Input: part model. Units: mm. Frame: model coordinates. Face numbers are marked on the shaded views. A direction names the side the tool comes from. Round coordinates to 2 decimals unless told otherwise and drop trailing zeros. Loops run counter-clockwise (first coordinate to the right, second up) from the corner with the lowest first, then second, coordinate; pieces in that order, holes last.
1) Access query for the marked faces 4 and 5. Directions: +Z, -Z, +X, -X, +Y, -Y. A direction counts if a zero-diameter tool reaches every point of the face in a straight line with its end or side. Return the directions, or none.
2) Ray query, line 1 along Y through (x, z) = (33, 70); line 2 along X through (y, z) = (22, 67.5); line 3 along Z through (x, y) = (37.5, 10.5). Return the intervals inside material, ascending.
3) Section C-C, the plane y = 71.5. Return loops of the section in (x, z).
4) Section A-A, the plane z = 45.5. Return loops of the section in (x, y), and give its area (3 significant figures).
5) Section B-B, the plane x = 59. Return loops of the section in (y, z).
6) Draft query along Y for the marked faces 1, 2 and 3. Return one class per face: pulls with the +Y half, pulls with the -Y half, needs draft (parallel to the pull), parting line crosses it, or undercut.
7) First-contact query: pin 1 (6 mm diameter, centred on x = 82, y = 57, fed in from +Z). Flat tip, straight axial feed; report the tip coordinate or a pass-through.
from build123d import *

# Parameters (mm, degrees)
SKETCH1_W           = 106.68
SKETCH1_H           = 81.28
BOSS_EXTRUDE1_DEPTH = 81.28
CHAMFER1_SIZE       = 15
SHELL2_T            = -6


with BuildPart() as part:
    # Sketch1 → Boss-Extrude1 (new body)
    with BuildSketch(Plane.XY):
        with Locations((53.34, 40.64)):
            Rectangle(SKETCH1_W, SKETCH1_H)
    extrude(amount=BOSS_EXTRUDE1_DEPTH)

    # Chamfer1
    chamfer1_edges = [part.edges().sort_by_distance(p)[0] for p in [
        (0, 81.28, 40.64),
        (106.68, 0, 40.64),
    ]]
    chamfer(chamfer1_edges, length=CHAMFER1_SIZE)

    # Shell2
    shell2_openings = [part.faces().sort_by_distance(p)[0] for p in [
        (53.34, 40.64, 81.28),
    ]]
    offset(amount=SHELL2_T, openings=shell2_openings, kind=Kind.INTERSECTION)


solid = part.part
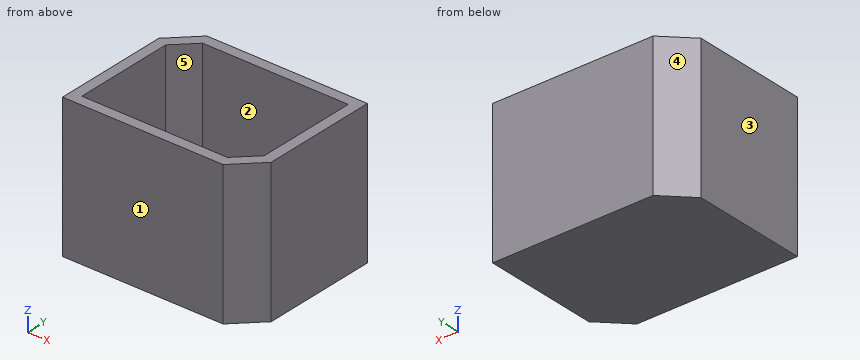
Final values:
1. face 4: +Z, -Z, -X, +Y
1. face 5: +Z
2. line 1: y = 0 to 6, 75.28 to 81.28
2. line 2: x = 0 to 6, 100.68 to 106.68
2. line 3: z = 0 to 6
3. outline: (5.22, 0) - (106.68, 0) - (106.68, 81.28) - (100.68, 81.28) - (100.68, 6) - (13.71, 6) - (13.71, 81.28) - (5.22, 81.28) - close
4. outline: (0, 0) - (91.68, 0) - (106.68, 15) - (106.68, 81.28) - (15, 81.28) - (0, 66.28) - close; hole (6, 6) - (89.19, 6) - (100.68, 17.49) - (100.68, 75.28) - (17.49, 75.28) - (6, 63.79) - close
4. area: 2,020 mm2
5. outline: (0, 0) - (81.28, 0) - (81.28, 81.28) - (75.28, 81.28) - (75.28, 6) - (6, 6) - (6, 81.28) - (0, 81.28) - close
6. face 1: pulls with the -Y half
6. face 2: undercut
6. face 3: needs draft
7. pin 1: stops at z = 6
